from build123d import *

# Parameters (mm, degrees)
SKETCH1_W               = 25
SKETCH1_H               = 5
BOSS_EXTRUDE2_DEPTH     = 30
CUT_EXTRUDE1_DEPTH      = 40.37003937
CUT_EXTRUDE1_DEPTH_BACK = 40.37003937
SKETCH2_R               = 2.5
SKETCH5_W               = 20
SKETCH5_H               = 5
BOSS_EXTRUDE3_DEPTH     = 20
CUT_EXTRUDE3_DEPTH      = 40.37003937


with BuildPart() as part:
    # Sketch1 → Boss-Extrude2 (new body)
    with BuildSketch(Plane.XY):
        with Locations((12.5, 2.5)):
            Rectangle(SKETCH1_W, SKETCH1_H)
    extrude(amount=BOSS_EXTRUDE2_DEPTH)

    # Sketch2 → Cut-Extrude1 (cut, two sides: drawn at the far end of the back side and taken through both)
    with BuildSketch(Plane(origin=(0, 5, 0), x_dir=(1, 0, 0), z_dir=(0, 1, 0)).offset(-CUT_EXTRUDE1_DEPTH_BACK)):
        with Locations(Location((6, -6, 0), (0, 0, 180))):
            Circle(SKETCH2_R)
        with Locations(Location((19, -6, 0), (0, 0, 180))):
            Circle(SKETCH2_R)
        with Locations(Location((19, -24, 0), (0, 0, 180))):
            Circle(SKETCH2_R)
        with Locations(Location((6, -24, 0), (0, 0, 180))):
            Circle(SKETCH2_R)
    extrude(amount=CUT_EXTRUDE1_DEPTH + CUT_EXTRUDE1_DEPTH_BACK, mode=Mode.SUBTRACT)

    # Sketch5 → Boss-Extrude3 (add)
    with BuildSketch(Plane.ZY):
        with Locations((15, 2.5)):
            Rectangle(SKETCH5_W, SKETCH5_H)
    extrude(amount=BOSS_EXTRUDE3_DEPTH)

    # Sketch6 → Cut-Extrude3 (cut, through all)
    with BuildSketch(Plane(origin=(0, 5, 0), x_dir=(1, 0, 0), z_dir=(0, 1, 0))):
        with BuildLine():
            Line((-12.044559796, -13.5), (-9.044559796, -13.5))
            Line((-9.044559796, -13.5), (-9.044559796, -16.5))
            Line((-9.044559796, -16.5), (-12.044559796, -16.5))
            ThreePointArc((-12.044559796, -16.5), (-14.044559796, -17.5), (-16.044559796, -16.5))
            Line((-16.044559796, -16.5), (-19.044559796, -16.5))
            Line((-19.044559796, -16.5), (-19.044559796, -13.5))
            Line((-19.044559796, -13.5), (-16.044559796, -13.5))
            ThreePointArc((-16.044559796, -13.5), (-14.044559796, -12.5), (-12.044559796, -13.5))
        make_face()
    extrude(amount=-CUT_EXTRUDE3_DEPTH, mode=Mode.SUBTRACT)


solid = part.part
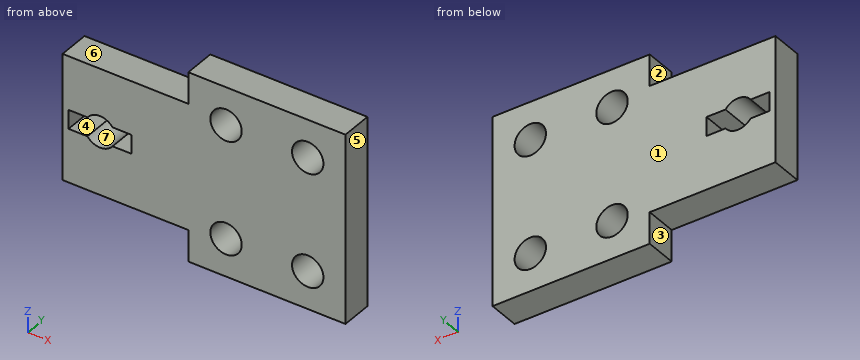
Design review of the part built by this model. Coordinates are the model's own, in mm. Face numbers are marked on the shaded views. A direction names the side the tool comes from. Coordinates: 2 decimals unless noted, no trailing zeros. Order: outer loops, then holes, each group sorted by start corner. A loop starts at its lowest first (then second) coordinate and runs counter-clockwise, first axis right, second up.
Item 1: For the marked faces 1, 2, 3 and 4, list the 3-axis set-ups (+Z, -Z, +X, -X, +Y, -Y) from which the entire face can be reached by the end or side of a thin tool; tool diameter is ignored.
Item 2: Take a section at C-C, the plane y = 4.2. Write out the cut boundary in (x, z), then the cut area to 3 significant figures.
Item 3: The part is to be moulded in two halves that separate along Z. For the marked faces 5, 6 and 7, say which applies: pulls with the +Z half, pulls with the -Z half, needs draft (parallel to the pull), parting line crosses it, or undercut.
Item 4: Take a section at A-A, the plane x = 6. Write out the cut boundary in (y, z), then the cut area to 3 significant figures.
Item 5: Take a section at D-D, the plane x = -5. Write out the cut boundary in (y, z).
Item 6: Take a section at B-B, the plane z = 4. Write out the cut boundary in (x, y), then the cut area to 3 significant figures.
Item 7: For line 1 (X direction, y = 3.25, z = 24); line 2 (Z direction, x = 19, y = 3.1); line 3 (X direction, y = 3.6, z = 25.75), list the stretches that pass through material, from the lowest coordinate up.
Item 8: For pin 1 Ø1.5 at (x, y) = (-18, 1.5) entering from +Z; pin 2 Ø2.5 at (y, z) = (3.5, 2) entering from -X; pin 3 Ø2.5 at (x, y) = (-10, 2.5) entering from -Z, all flat-tipped, find the tip position at first contact; note any pin that passes through.
The answers:
1. face 1: +Z, -Z, +X, -X, +Y
1. face 2: +Z, -X, +Y, -Y
1. face 3: -Z, -X, +Y, -Y
1. face 4: +Y, -Y
2. outline: (-20, 5) - (0, 5) - (0, 0) - (25, 0) - (25, 30) - (0, 30) - (0, 25) - (-20, 25) - close; hole (-19.04, 13.5) - (-16.04, 13.5) arc R2.5 ccw to (-12.04, 13.5) - (-9.04, 13.5) - (-9.04, 16.5) - (-12.04, 16.5) arc R2.5 ccw to (-16.04, 16.5) - (-19.04, 16.5) - close; hole circle Ø5 at (6, 6); hole circle Ø5 at (6, 24); hole circle Ø5 at (19, 6); hole circle Ø5 at (19, 24)
2. area: 1,040 mm2
3. face 5: needs draft
3. face 6: pulls with the +Z half
3. face 7: undercut
4. outline: (0, 0) - (5, 0) - (5, 3.5) - (0, 3.5) - close; (0, 8.5) - (5, 8.5) - (5, 21.5) - (0, 21.5) - close; (0, 26.5) - (5, 26.5) - (5, 30) - (0, 30) - close
4. area: 100 mm2
5. outline: (0, 5) - (5, 5) - (5, 25) - (0, 25) - close
6. outline: (0, 0) - (4.5, 0) - (4.5, 5) - (0, 5) - close; (7.5, 0) - (17.5, 0) - (17.5, 5) - (7.5, 5) - close; (20.5, 0) - (25, 0) - (25, 5) - (20.5, 5) - close
6. area: 95.0 mm2
7. line 1: x = -20 to 3.5, 8.5 to 16.5, 21.5 to 25
7. line 2: z = 0 to 3.5, 8.5 to 21.5, 26.5 to 30
7. line 3: x = 0 to 4.21, 7.79 to 17.21, 20.79 to 25
8. pin 1: stops at z = 25
8. pin 2: stops at x = 0
8. pin 3: stops at z = 5
